Input: part model. Units: mm. Frame: model coordinates. Coordinates: 2 decimals unless noted, no trailing zeros. Order: outer loops, then holes, each group sorted by start corner. A loop starts at its lowest first (then second) coordinate and runs counter-clockwise, first axis right, second up. Notation, with made-up numbers: (25, -11.5) - (58, -11.5) arc R26 cw to (58, 26.5) - close; hole circle Ø1 at (-27.75, 62). An arc over 180 degrees is marked (long way). Answer as CSV lines item,"result". Start each with the question number.
Item 1: Section A-A (y = -22.5). Output: boundary loops of the cut face in (x, z) (1 decimal), and give its area (3 significant figures).
Item 2: Section C-C (x = 2). Output: boundary loops of the cut face in (y, z), and give its area (3 significant figures).
Item 3: First-contact query: pin 1 (10 mm diameter, centred on y = -27.5, z = -12, fed in from -X); pin 2 (3 mm diameter, centred on x = -10, y = -19.5, fed in from +Z); pin 3 (5 mm diameter, centred on y = -20, z = -11, fed in from -X); pin 4 (4 mm diameter, centred on x = -11, z = 3, fed in from -Y). Flat tips, straight axial feed; report the tip coordinate or a pass-through.
Item 4: Section B-B (z = -14). Output: boundary loops of the cut face in (x, y), and give its area (3 significant figures).
Item 5: Material intervals for line 1 along X through (y, z) = (-5, 7.75); line 2 along X through (y, z) = (-12, -12.75); line 3 along Z through (x, y) = (8.5, -17), sorted ascending.
from build123d import *

# Parameters (mm, degrees)
F1_DEPTH = 38.1


with BuildPart() as f1:
    # F0 (on Front) → F1 (new body)
    with BuildSketch(Plane.XZ):
        with BuildLine():
            Line((-4.0410087584, -2.3330774944), (0, 0))
            Line((0, 0), (0, 4.6661549889))
            ThreePointArc((0, 4.6661549889), (-7.8066293313, 5.6939172222), (-15.0812497909, 8.7071636265))
            ThreePointArc((-15.0812497909, 8.7071636265), (-8.8343916271, 3.9137807077), (-4.0410087584, -2.3330774944))
        make_face()
        with BuildLine():
            Line((0, 0), (4.0410087584, -2.3330774944))
            ThreePointArc((4.0410087584, -2.3330774944), (8.8343919533, 3.913781034), (15.0812505899, 8.7071640878))
            ThreePointArc((15.0812505899, 8.7071640878), (7.8066297769, 5.6939173416), (0, 4.6661549889))
            Line((0, 4.6661549889), (0, 0))
        make_face()
        with BuildLine():
            ThreePointArc((0, -17.4143274944), (1.0277622646, -9.6076980465), (4.0410087584, -2.3330774944))
            Line((4.0410087584, -2.3330774944), (0, 0))
            Line((0, 0), (-4.0410087584, -2.3330774944))
            ThreePointArc((-4.0410087584, -2.3330774944), (-1.0277622646, -9.6076980465), (0, -17.4143274944))
        make_face()
    extrude(amount=F1_DEPTH)


solid = f1.part
Determined:
1,outline,"(-15.1, 8.7) arc R30.2 cw to (0, -17.4) arc R30.2 cw to (15.1, 8.7) arc R30.2 cw to start"
1,area,"147 mm^2"
2,outline,"(-38.1, -6.61) - (0, -6.61) - (0, 4.73) - (-38.1, 4.73) - close"
2,area,"432 mm^2"
3,pin 1,"stops at x = -1.85"
3,pin 2,"stops at z = 6.94"
3,pin 3,"stops at x = -1.35"
3,pin 4,"passes through"
4,outline,"(-0.19, -38.1) - (0.19, -38.1) - (0.19, 0) - (-0.19, 0) - close"
4,area,"14.8 mm^2"
5,line 1,"x = -13.53 to -13.29, 13.29 to 13.53"
5,line 2,"x = -0.36 to 0.36"
5,line 3,"z = 3.57 to 5.89"
